For this review, take the finished solid that the model builds, in its own axes (mm). Face numbers are marked on the shaded views. A direction names the side the tool comes from. Give positions to 0.01 mm unless a question says otherwise; leave off trailing zeros. Write each loop counter-clockwise with the first axis right and the second up, starting at its lowest first coordinate (ties: lowest second). Pieces come first, ordered by that corner, then holes.
Q1. We need section C-C (y = 27.5). Write out the cut boundary in (x, z).
Q2. We need section B-B (x = 0). Write out the cut boundary in (y, z), then the cut area to 3 significant figures.
Q3. Insertion check: P1, Ø12, axis at x = -18.5, y = 17.5, coming from the +Z side; P2, Ø2.5, axis at x = 18.5, y = 28, coming from the +Z side; P3, Ø3, axis at x = -10.5, y = 25.5, coming from the -Z side; P4, Ø3, axis at x = -6.5, z = -16, coming from the -Y side. Each pin has a flat end and moves straight along its axis. Give the tip position at first contact, or say it passes through.
Q4. Machinability: for the marked faces 1 and 2, which of the approach directions +Z, -Z, +X, -X, +Y, -Y give a long, thin tool a straight path to every point of the face, cutting with its end or side? Answer none if there is none.
Q5. We need section A-A (z = 0). Write out the cut boundary in (x, y).
Q6. We need section D-D (y = 8.25). Write out the cut boundary in (x, z), then the cut area to 3 significant figures.
Q7. Mouldability with a two-part tool opening along Z and no side actions: class the marked faces 3, 4 and 5 as released by +Z, released by -Z, zero draft, split by the parting line, or undercut.
Q8. For line 1 (Y direction, x = -11, z = 2.5); line 2 (X direction, y = 6.25, z = 2), list the stretches that pass through material, from the lowest coordinate up.
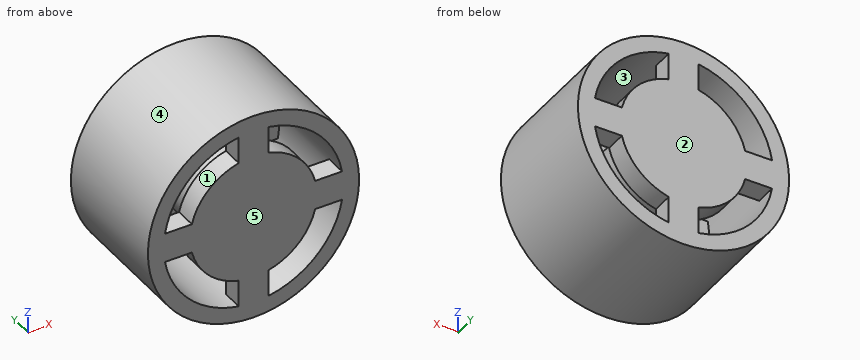
Autodesk Inventor part; units mm, degrees
ref_plane "YZ Plane" through (0, 0, 0) normal (1, 0, 0) x (0, 1, 0)
ref_plane "XZ Plane" through (0, 0, 0) normal (0, 1, 0) x (-1, 0, 0)
ref_plane "XY Plane" through (0, 0, 0) normal (0, 0, 1) x (1, 0, 0)
sketch "Sketch1" plane through (0, 0, 0) normal (0, 1, 0) x (-1, 0, 0)
  circle A0 centre (0, 0) radius 25
  dimension "d0" = 50
extrude "Extrusion1" add sketch "Sketch1" along normal blind 30
sketch "Sketch2" plane through (0, 30, 0) normal (0, 1, 0) x (1, 0, 0)
  circle A0 centre (0, 0) radius 21.25
  dimension "d3" = 42.5
extrude "Extrusion2" cut sketch "Sketch2" against normal blind 30
sketch "Sketch3" plane through (0, 30, 0) normal (0, 1, 0) x (1, 0, 0)
  circle A0 centre (0, 0) radius 15
  dimension "d6" = 30
extrude "Extrusion3" add sketch "Sketch3" against normal blind 5
sketch "Sketch4" plane through (0, 30, 0) normal (0, 1, 0) x (1, 0, 0)
  circle A0 centre (0, 0) radius 21.25
  line L0 (0, -12.25) -> (3.5, -12.25)
  line L1 (3.5, -12.25) -> (3.5, -22.5574)
  line L2 (3.5, -22.5574) -> (-3.5, -22.5574)
  line L3 (-3.5, -22.5574) -> (-3.5, -12.25)
  line L4 (-3.5, -12.25) -> (0, -12.25)
  point P0 (-3.5, -20.9598)
  point P1 (3.5, -20.9598)
  dimension "d10" = 3.5
  dimension "d11" = 7
extrude "Extrusion4" add sketch "Sketch4" against normal blind 5 contours L3 L4 L0 L1 A0 picked at (1.5571, -15.2392)
sketch "Sketch5" plane through (0, 30, 0) normal (0, 1, 0) x (1, 0, 0)
  circle A0 centre (0, 0) radius 21.25
  line L0 (12.1299, 0) -> (12.1299, 3.5)
  line L1 (12.1299, 3.5) -> (23.3023, 3.5)
  line L2 (23.3023, 3.5) -> (23.3023, -3.5)
  line L3 (23.3023, -3.5) -> (12.1299, -3.5)
  line L4 (12.1299, -3.5) -> (12.1299, 3.5)
  point P0 (20.9598, -3.5)
  point P1 (20.9598, 3.5)
  dimension "d16" = 3.5
  dimension "d17" = 7
extrude "Extrusion5" add sketch "Sketch5" against normal blind 5 contours A0 L3 L4 L0 L1 picked at (15.1269, -1.9464)
sketch "Sketch6" plane through (0, 30, 0) normal (0, 1, 0) x (1, 0, 0)
  line L0 (0, 13.5132) -> (-3.5, 13.5132)
  line L1 (-3.5, 13.5132) -> (-3.5, 23.3023)
  line L2 (-3.5, 23.3023) -> (3.5, 23.3023)
  line L3 (3.5, 23.3023) -> (3.5, 13.5132)
  line L4 (3.5, 13.5132) -> (-3.5, 13.5132)
  point P0 (0, 0)
  dimension "d20" = 7
extrude "Extrusion6" add sketch "Sketch6" against normal blind 5
sketch "Sketch7" plane through (0, 30, 0) normal (0, 1, 0) x (1, 0, 0)
  line L0 (-12.9812, 0) -> (-12.9812, -3.5)
  line L1 (-12.9812, -3.5) -> (-22.5574, -3.5)
  line L2 (-22.5574, -3.5) -> (-22.5574, 3.5)
  line L3 (-22.5574, 3.5) -> (-12.9812, 3.5)
  line L4 (-12.9812, 3.5) -> (-12.9812, 0)
  point P0 (0, 0)
  dimension "d23" = 3.5
  dimension "d24" = 7
extrude "Extrusion7" add sketch "Sketch7" against normal blind 5
sketch "Sketch8" plane through (0, 25, 0) normal (0, -1, 0) x (1, 0, 0)
  circle A0 centre (0, 0) radius 10
  dimension "d27" = 20
extrude "Extrusion8" add sketch "Sketch8" along normal blind 20
sketch "Sketch9" plane through (0, 5, 0) normal (0, -1, 0) x (1, 0, 0)
  circle A0 centre (0, 0) radius 7.5
  dimension "d30" = 15
extrude "Extrusion9" cut sketch "Sketch9" against normal blind 20
sketch "Sketch10" plane through (0, 0, 0) normal (0, -1, 0) x (1, 0, 0)
  circle A0 centre (0, 0) radius 15
extrude "Extrusion10" add sketch "Sketch10" against normal blind 5
sketch "Sketch11" plane through (0, 0, 0) normal (0, -1, 0) x (1, 0, 0)
  line L0 (12.662, 0) -> (12.662, 3.5)
  line L1 (12.662, 3.5) -> (22.2382, 3.5)
  line L2 (22.2382, 3.5) -> (22.2382, -3.5)
  line L3 (22.2382, -3.5) -> (12.662, -3.5)
  line L4 (12.662, -3.5) -> (12.662, 0)
  point P0 (0, 0)
  dimension "d35" = 3.5
  dimension "d36" = 7
extrude "Extrusion11" add sketch "Sketch11" against normal blind 5
sketch "Sketch12" plane through (0, 0, 0) normal (0, -1, 0) x (1, 0, 0)
  line L0 (0, 12.3428) -> (3.5, 12.3428)
  line L1 (3.5, 12.3428) -> (3.5, 22.5574)
  line L2 (3.5, 22.5574) -> (-3.5, 22.5574)
  line L3 (-3.5, 22.5574) -> (-3.5, 12.3428)
  line L4 (-3.5, 12.3428) -> (0, 12.3428)
  point P0 (0, 0)
  dimension "d39" = 3.5
  dimension "d40" = 7
extrude "Extrusion12" add sketch "Sketch12" against normal blind 5
sketch "Sketch13" plane through (0, 0, 0) normal (0, -1, 0) x (1, 0, 0)
  line L0 (0, -13.726) -> (3.5, -13.726)
  line L1 (3.5, -13.726) -> (3.5, -22.5574)
  line L2 (3.5, -22.5574) -> (-3.5, -22.5574)
  line L3 (-3.5, -22.5574) -> (-3.5, -13.726)
  line L4 (-3.5, -13.726) -> (0, -13.726)
  point P0 (0, 0)
  dimension "d43" = 3.5
  dimension "d44" = 7
extrude "Extrusion13" add sketch "Sketch13" against normal blind 5
sketch "Sketch14" plane through (0, 0, 0) normal (0, -1, 0) x (1, 0, 0)
  line L0 (-12.0235, 0) -> (-12.0235, -3.5)
  line L1 (-12.0235, -3.5) -> (-22.451, -3.5)
  line L2 (-22.451, -3.5) -> (-22.451, 3.5)
  line L3 (-22.451, 3.5) -> (-12.0235, 3.5)
  line L4 (-12.0235, 3.5) -> (-12.0235, 0)
  point P0 (0, 0)
  dimension "d47" = 3.5
  dimension "d48" = 7
extrude "Extrusion14" add sketch "Sketch14" against normal blind 5
properties part number "Wheel"
Computed:
1. outline: circle Ø50 at (0, 0); hole (-20.96, -3.5) arc R21.25 ccw to (-3.5, -20.96) - (-3.5, -14.59) arc R15 cw to (-14.59, -3.5) - close; hole (-20.96, 3.5) - (-14.59, 3.5) arc R15 cw to (-3.5, 14.59) - (-3.5, 20.96) arc R21.25 ccw to start; hole (3.5, -20.96) arc R21.25 ccw to (20.96, -3.5) - (14.59, -3.5) arc R15 cw to (3.5, -14.59) - close; hole (3.5, 14.59) arc R15 cw to (14.59, 3.5) - (20.96, 3.5) arc R21.25 ccw to (3.5, 20.96) - close
2. outline: (0, -25) - (30, -25) - (30, 25) - (0, 25) - close; hole (5, -21.25) - (25, -21.25) - (25, -10) - (5, -10) - close; hole (5, -7.5) - (25, -7.5) - (25, 7.5) - (5, 7.5) - close; hole (5, 10) - (25, 10) - (25, 21.25) - (5, 21.25) - close
2. area: 750 mm2
3. P1: stops at z = 21.65
3. P2: stops at z = 18.1
3. P3: stops at z = -23.32
3. P4: passes through
4. face 1: +Y, -Y
4. face 2: +Z, -Z, +X, -X, +Y
5. outline: (-25, 0) - (25, 0) - (25, 30) - (-25, 30) - close; hole (-21.25, 5) - (-10, 5) - (-10, 25) - (-21.25, 25) - close; hole (-7.5, 5) - (7.5, 5) - (7.5, 25) - (-7.5, 25) - close; hole (10, 5) - (21.25, 5) - (21.25, 25) - (10, 25) - close
6. outline: circle Ø50 at (0, 0); circle Ø20 at (0, 0); hole circle Ø42.5 at (0, 0); hole circle Ø15 at (0, 0)
6. area: 682 mm2
7. face 3: undercut
7. face 4: split by the parting line
7. face 5: zero draft
8. line 1: y = 0 to 5, 25 to 30
8. line 2: x = -24.92 to -21.16, -9.8 to -7.23, 7.23 to 9.8, 21.16 to 24.92
